Autodesk Inventor part; units mm, degrees
ref_plane "YZ Plane" through (0, 0, 0) normal (1, 0, 0) x (0, 1, 0)
ref_plane "XZ Plane" through (0, 0, 0) normal (0, 1, 0) x (-1, 0, 0)
ref_plane "XY Plane" through (0, 0, 0) normal (0, 0, 1) x (1, 0, 0)
sketch "Sketch1" plane through (0, 0, 0) normal (0, 1, 0) x (-1, 0, 0)
  line L0 (0, -140) -> (0, 140)
  line L1 (-350, 0) -> (350, 0)
  line L2 (-250, 100) -> (-250, -100)
  line L3 (-250, -100) -> (250, -100)
  line L4 (250, -100) -> (250, 100)
  line L5 (250, 100) -> (175, 100)
  line L6 (175, 100) -> (175, -50)
  line L7 (175, -50) -> (-200, -50)
  line L8 (-200, -50) -> (-200, 100)
  line L9 (-200, 100) -> (-250, 100)
  dimension "d0" = 200
  dimension "d1" = 50
  dimension "d2" = 50
  dimension "d3" = 500
  dimension "d4" = 75
extrude "Extrusion1" add sketch "Sketch1" along normal mid plane 250 contours L3 L2 L1 L8 L7 L0 | L0 L7 L6 L1 L4 L3 | L2 L9 L8 L1 | L1 L6 L5 L4
fillet "Fillet1" radius 75 1 edges at (250, 0, -100)
fillet "Fillet1" radius 25 1 edges at (200, 0, -50)
sketch "Sketch2" plane through (-250, 125, 100) normal (0, 0, 1) x (1, 0, 0)
  line L0 (0, -250) -> (0, 0)
  line L1 (0, -250) -> (75, -250)
  line L2 (75, -250) -> (75, 0)
  circle A0 centre (37.5, -212.5) radius 37.5 construction
  circle A1 centre (37.5, -212.5) radius 20
  dimension "d9" = 40
extrude "Extrusion2" add sketch "Sketch2" along normal blind 50
sketch "Sketch3" plane through (200, 125, 100) normal (0, 0, 1) x (1, 0, 0)
  line L0 (0, -250) -> (50, -250)
  circle A0 centre (-412.5, -212.5) radius 20
  circle A1 centre (25, -212.5) radius 15
  point P0 (25, -250)
  dimension "d12" = 30
extrude "Extrusion3" add sketch "Sketch3" along normal up to surface (50 mm away) contours A1
sketch "Sketch4" plane through (0, 0, 0) normal (0, 1, 0) x (-1, 0, 0)
  line L0 (-175, -50) -> (175, -50)
  line L1 (-12.5, -50) -> (12.5, -50)
  line L2 (12.5, -50) -> (12.5, 50)
  line L3 (12.5, 50) -> (-12.5, 50)
  line L4 (-12.5, 50) -> (-12.5, -50)
  line L5 (0, -150) -> (0, 200)
  dimension "d15" = 25
  dimension "d16" = 100
extrude "Extrusion4" add sketch "Sketch4" along normal mid plane 175
sketch "Sketch5" plane through (-175, -125, 100) normal (1, 0, 0) x (0, 0, -1)
  circle A0 centre (7.5, 125) radius 7.5
  line L0 (0, 250) -> (0, 0)
  point P0 (0, 125)
  dimension "d19" = 15
extrude "Extrusion5" add sketch "Sketch5" along normal up to next
properties part number "Interactice Exercise"
Source: CAD feature listing. Evaluate the final solid. Frame: model axes, mm. A direction names the side the tool comes from. Give positions to 0.01 mm unless a question says otherwise; leave off trailing zeros. Write each loop counter-clockwise with the first axis right and the second up, starting at its lowest first coordinate (ties: lowest second). Pieces come first, ordered by that corner, then holes. Notation, with made-up numbers: (-39.5, 5.5) -> (-9.5, 5.5) arc R10 cw to (-9.5, 22.5) -> close; hole circle Ø5 at (32, 40.5). An arc over 180 degrees is marked (long way). Write item = value, one per line.
Q1. Cut plane A-A on z = 44. Return loops of the section in (x, y), then the cut area to 3 significant figures.
Here are the results:
outline = (-250, -125) -> (-175, -125) -> (-175, 125) -> (-250, 125) -> close; (-12.5, -87.5) -> (12.5, -87.5) -> (12.5, 87.5) -> (-12.5, 87.5) -> close; (200, -125) -> (250, -125) -> (250, 125) -> (200, 125) -> close
area = 35,600 mm²
Q2. Cut plane D-D on z = 92.5. Return loops of the section in (x, y), then the cut area to 3 significant figures.
Here are the results:
outline = (-250, -125) -> (-175, -125) -> (-175, -7.5) -> (200, -7.5) -> (200, -125) -> (250, -125) -> (250, 125) -> (200, 125) -> (200, 7.5) -> (-175, 7.5) -> (-175, 125) -> (-250, 125) -> close
area = 36,900 mm²
Q3. Cut plane C-C on x = -212.5. Return loops of the section in (y, z).
Here are the results:
outline = (-125, -100) -> (125, -100) -> (125, 100) -> (-67.5, 100) -> (-67.5, 150) -> (-107.5, 150) -> (-107.5, 100) -> (-125, 100) -> close
Q4. First-contact query: pin 1 (12.5 mm diameter, centred on x = -5, y = -17, fed in from +Z); pin 2 (5 mm diameter, centred on x = 103, y = -10.5, fed in from +Z); pin 3 (25 mm diameter, centred on x = 214, y = 26.5, fed in from +Z). Flat tips, straight axial feed; report the tip coordinate or a pass-through.
Here are the results:
pin_1 = 50
pin_2 = -50
pin_3 = 100
Q5. Line query: line 1 (X direction, y = -37, z = -18.5); line 2 (X direction, y = 40.5, z = 55); line 3 (X direction, y = 33, z = -36.5). Output: solid intervals per line, ascending. Write a range as from..to.
Here are the results:
line_1 = -250..-175, -12.5..12.5, 200..250
line_2 = -250..-175, 200..250
line_3 = -250..-175, -12.5..12.5, 197.2..249.11
Q6. Reachability of faces 1 (the face through (238.856, -81.755, 124.65)), 2 (the face through (10, 0, 100)), 3 (the face through (0, -87.5, 1)), 4 (the face through (0, 87.5, 1)) from +Z, -Z, +X, -X, +Y, -Y: full face, straight path, thin tool, end or side. Return the list, or none.
Here are the results:
face_1 = +Z
face_2 = none
face_3 = +Z, -Y
face_4 = +Z, +Y
Q7. Mould query, pull axis X, two halves, no side actions, for faces 5 (the face through (-213, -87, 150)), 6 (the face through (250, -2, 38)), 7 (the face through (-12.5, -1, -1)), 8 (the face through (-228.37, -75.33, 124.65)). Classes: +X half, -X half, draft (parallel to the pull), parting line (faces both ways), or undercut.
Here are the results:
face_5 = draft
face_6 = +X half
face_7 = undercut
face_8 = undercut
Q8. Cut plane B-B on y = 69. Return loops of the section in (x, z).
Here are the results:
outline = (-250, -100) -> (175, -100) arc R75 ccw to (250, -25) -> (250, 100) -> (200, 100) -> (200, -25) arc R25 cw to (175, -50) -> (12.5, -50) -> (12.5, 50) -> (-12.5, 50) -> (-12.5, -50) -> (-175, -50) -> (-175, 100) -> (-250, 100) -> close
